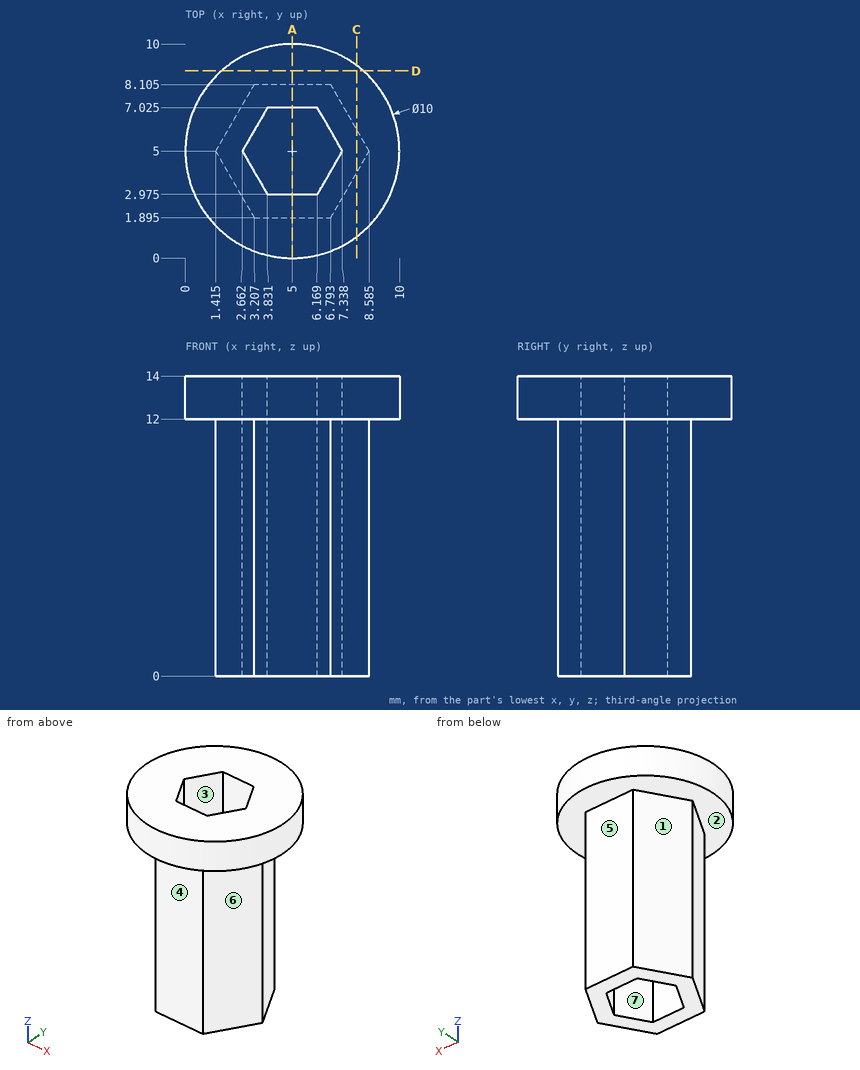
Part print with two shaded views. Sizes in mm from the minimum x, y, z corner. A direction names the side the tool comes from. Give positions to 0.01 mm unless a question says otherwise; leave off trailing zeros. Loops run counter-clockwise (first coordinate to the right, second up) from the corner with the lowest first, then second, coordinate; pieces in that order, holes last. Notation, with made-up numbers: (-12.75, -2.5) - (-1.75, -2.5) arc R34 ccw to (-1.75, 29.5) - close; hole circle Ø7 at (84, 46.5). An arc over 180 degrees is marked (long way). Put each result on its own line as item: value.
Q1. Flat gauge pins, fed straight in: pin 1 (5 mm diameter, centred on y = 4.5, z = 2, fed in from +X) (1 decimal); pin 2 (3 mm diameter, centred on x = 5.5, z = 5.5, fed in from -Y) (3 decimals); pin 3 (3 mm diameter, centred on x = 1, z = 9.5, fed in from +Y). Where does each tip first touch, or does it go through?
Filled in:
pin 1: stops at x = 8.6
pin 2: stops at y = 1.895
pin 3: stops at y = 6.88
Q2. Mould opens along Y. For the marked faces 1, 2, 3 and 4 say: pulls with the +Y half, pulls with the -Y half, needs draft (parallel to the pull), parting line crosses it, or undercut.
Filled in:
face 1: pulls with the +Y half
face 2: needs draft
face 3: undercut
face 4: pulls with the -Y half
Q3. Slice it at A-A (x = 5). Give the cut face in (y, z) (1 decimal).
Filled in:
outline: (0, 12) - (1.9, 12) - (1.9, 0) - (3, 0) - (3, 14) - (0, 14) - close; (7, 0) - (8.1, 0) - (8.1, 12) - (10, 12) - (10, 14) - (7, 14) - close
Q4. Slice it at D-D (y = 8.75). Give the cut face in (x, z).
Filled in:
outline: (1.69, 12) - (8.31, 12) - (8.31, 14) - (1.69, 14) - close
Q5. Probe line 1 along Y through (x, z) = (5.25, 11.25) (1 decimal); line 2 along Z through (x, y) = (1.5, 2.5); line 3 along Y through (x, z) = (3, 7.25) (1 decimal). List the from-to ranges inside material, lowest first.
Filled in:
line 1: y = 1.9 to 3, 7 to 8.1
line 2: z = 12 to 14
line 3: y = 2.3 to 4.4, 5.6 to 7.7
Q6. Slice it at C-C (x = 8). Give the cut face in (y, z).
Filled in:
outline: (1, 12) - (3.99, 12) - (3.99, 0) - (6.01, 0) - (6.01, 12) - (9, 12) - (9, 14) - (1, 14) - close
Q7. Tool access for the marked faces 5, 6 and 7: list every direction of +Z, -Z, +X, -X, +Y, -Y with a clear straight run to the whole face (end or side of a thin tool).
Filled in:
face 5: -Z, +X, -X, +Y
face 6: -Z, +X, -Y
face 7: +Z, -Z
